Can you work these out from the model? Positions are in its coordinate system, mm. Coordinates: 2 decimals unless noted, no trailing zeros. Loops run counter-clockwise (first coordinate to the right, second up) from the corner with the lowest first, then second, coordinate; pieces in that order, holes last.
```python
from build123d import *

# Parameters (mm, degrees)
F0_R          = 35
F0_R_2        = 20
F1_DEPTH      = 3.5
F2_R          = 1.5
F4_DEPTH      = 35.001
F4_DEPTH_BACK = 35.001
F3_R          = 1.5
F5_DEPTH      = 35.0010001
F5_DEPTH_BACK = 35.0010001


with BuildPart() as f1:
    # F0 (on Top) → F1 (new body, symmetric)
    with BuildSketch(Plane.XY):
        Circle(F0_R)
        Circle(F0_R_2, mode=Mode.SUBTRACT)
    extrude(amount=F1_DEPTH, both=True)

    # F2 (on Right) → F4 (cut, two sides)
    with BuildSketch(Plane.YZ) as f4_sk:
        Circle(F2_R)
    extrude(amount=-F4_DEPTH, mode=Mode.SUBTRACT)
    extrude(f4_sk.sketch, amount=F4_DEPTH_BACK, mode=Mode.SUBTRACT)

    # F3 (on Front) → F5 (cut, two sides)
    with BuildSketch(Plane.XZ) as f5_sk:
        Circle(F3_R)
    extrude(amount=-F5_DEPTH, mode=Mode.SUBTRACT)
    extrude(f5_sk.sketch, amount=F5_DEPTH_BACK, mode=Mode.SUBTRACT)


solid = f1.part
```
(1) If we mould it in two halves opening along Y, with no side actions, what happens to faces 1 (the flat face through (15, -15, 3.5)), 2 (the cylindrical face through (-28, -21, 0)), 3 (the cylindrical face through (27.37, -1.5, 0.07))? For each: released by +Y, released by -Y, zero draft, split by the parting line, or undercut.
Check values:
face 1: zero draft
face 2: split by the parting line
face 3: undercut
(2) I'm going to push flat-ended pins straight in: pin 1 (3 mm diameter, centred on y = -4.5, z = 2.5, fed in from -X); pin 2 (1.5 mm diameter, centred on y = -20.5, z = -2.5, fed in from +X); pin 3 (2 mm diameter, centred on x = -19.5, z = -2, fed in from -Y). Where does each tip first touch, or does it pass through?
Check values:
pin 1: stops at x = -34.87
pin 2: stops at x = 28.9
pin 3: stops at y = -29.71
(3) I want a section at C-C on x = 30. Write out the boundary of the cut face in (y, z).
Check values:
outline: (-18.03, -3.5) - (18.03, -3.5) - (18.03, 3.5) - (-18.03, 3.5) - close; hole circle Ø3 at (0, 0)
(4) I want a section at D-D on y = -24. Write out the boundary of the cut face in (x, z), then the cut area to 3 significant figures.
Check values:
outline: (-25.48, -3.5) - (25.48, -3.5) - (25.48, 3.5) - (-25.48, 3.5) - close; hole circle Ø3 at (0, 0)
area: 350 mm2
(5) I want a section at A-A on x = 0. Write out the boundary of the cut face in (y, z).
Check values:
outline: (-35, -3.5) - (-20, -3.5) - (-20, -1.5) - (-35, -1.5) - close; (-35, 1.5) - (-20, 1.5) - (-20, 3.5) - (-35, 3.5) - close; (20, -3.5) - (35, -3.5) - (35, -1.5) - (20, -1.5) - close; (20, 1.5) - (35, 1.5) - (35, 3.5) - (20, 3.5) - close
(6) If I drill on probe 1 along Z at (x, y) = (0, -26); probe 2 along X at (y, z) = (-5.5, -0.25); probe 3 along Y at (x, z) = (12, 1.75), over which ranges is the centre line in solid material (lowest first)?
Check values:
probe 1: z = -3.5 to -1.5, 1.5 to 3.5
probe 2: x = -34.57 to -19.23, 19.23 to 34.57
probe 3: y = -32.88 to -16, 16 to 32.88
